from build123d import *

# Parameters (mm, degrees)
SKETCH_1_W        = 85
SKETCH_1_H        = 65
EXTRUDE_1_DEPTH   = 2.5
SKETCH_3_W        = 79.7
SKETCH_3_H        = 59.7
EXTRUDE_2_DEPTH   = 2.5
SHELL_START       = 2.5
SHELL_1_OUTLINE_W = 74.7
SHELL_1_OUTLINE_H = 54.7
SHELL_1_DEPTH     = 2.5


# Read off the part's stored shape, not the designer's step: 抽壳1
with BuildPart() as part:
    # 草图1 → 凸台-拉伸1 (new body)
    with BuildSketch(Plane(origin=(0, 0, 0), x_dir=(1, 0, 0), z_dir=(0, 1, 0))):
        Rectangle(SKETCH_1_W, SKETCH_1_H)
    extrude(amount=EXTRUDE_1_DEPTH)

    # 草图3 → 凸台-拉伸2 (add)
    with BuildSketch(Plane(origin=(0, 2.5, 0), x_dir=(1, 0, 0), z_dir=(0, 1, 0))):
        Rectangle(SKETCH_3_W, SKETCH_3_H)
    extrude(amount=EXTRUDE_2_DEPTH)

    # 抽壳1 outline → 抽壳1 (cut)
    with BuildSketch(Plane(origin=(0, 0, 0), x_dir=(1, 0, 0), z_dir=(0, 1, 0)).offset(SHELL_START)):
        Rectangle(SHELL_1_OUTLINE_W, SHELL_1_OUTLINE_H)
    extrude(amount=SHELL_1_DEPTH, mode=Mode.SUBTRACT)


solid = part.part
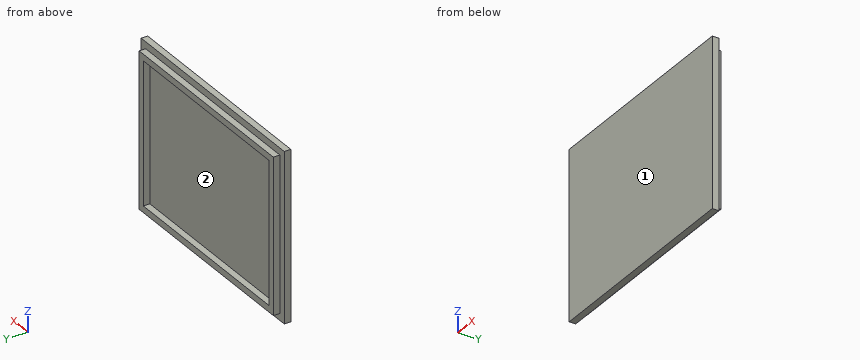
For this review, take the finished solid that the model builds, in its own axes (mm). Face numbers are marked on the shaded views. Round coordinates to 2 decimals unless told otherwise and drop trailing zeros. Order: outer loops, then holes, each group sorted by start corner. A loop starts at its lowest first (then second) coordinate and runs counter-clockwise, first axis right, second up. Notation, with made-up numbers: M 28.25,31 L 77.25,31 A25 ccw 77.25,43 Z; hole C -26,-13.75 d5. An arc over 180 degrees is marked long. Use a Markdown table: item, result. Add a question column.
Item 1: Insertion check: pin 1 (12 mm diameter, centred on x = -30, z = -20, fed in from +Y); pin 2 (1.5 mm diameter, centred on x = -8.5, y = 4, fed in from -Z); pin 3 (1.2 mm diameter, centred on x = -6.5, y = 4.5, fed in from +Z). Each pin has a flat end and moves straight along its axis. Give the tip position at first contact, or say it passes through.
Item 2: To check wall thickness, follow line 1 along X through (y, z) = (3.3, 26.5); line 2 along Z through (x, y) = (10.5, 4.3); line 3 along Y through (x, z) = (0, 21). State the ranges of each line that lie inside material, in increasing order.
Item 3: Mouldability with a two-part tool opening along X and no side actions: class the marked faces 1 and 2 as released by +X, released by -X, zero draft, split by the parting line, or undercut.
Item 4: Add section A-A, the plane z = -12. Give the boundary of the cut face in (x, y), then the cut area to 3 significant figures.
Item 5: Add section B-B, the plane x = -8. Give the boundary of the cut face in (y, z).
Geometry results:
| question | item | result |
|---|---|---|
| 1 | pin 1 | stops at y = 2.5 |
| 1 | pin 2 | stops at z = -29.85 |
| 1 | pin 3 | stops at z = 29.85 |
| 2 | line 1 | x = -39.85 to -37.35, 37.35 to 39.85 |
| 2 | line 2 | z = -29.85 to -27.35, 27.35 to 29.85 |
| 2 | line 3 | y = 0 to 2.5 |
| 3 | face 1 | zero draft |
| 3 | face 2 | undercut |
| 4 | outline | M -42.5,0 L 42.5,0 L 42.5,2.5 L 39.85,2.5 L 39.85,5 L 37.35,5 L 37.35,2.5 L -37.35,2.5 L -37.35,5 L -39.85,5 L -39.85,2.5 L -42.5,2.5 Z |
| 4 | area | 225 mm² |
| 5 | outline | M 0,-32.5 L 2.5,-32.5 L 2.5,-29.85 L 5,-29.85 L 5,-27.35 L 2.5,-27.35 L 2.5,27.35 L 5,27.35 L 5,29.85 L 2.5,29.85 L 2.5,32.5 L 0,32.5 Z |
